from build123d import *

# Parameters (mm, degrees)
CHAMFER1_SIZE  = 0.79375
CHAMFER1_SIZE2 = 0.458271776
FILLET1_R      = 0.396875


with BuildPart() as part:
    # Sketch1 → Revolve1 (revolve)
    with BuildSketch(Plane.XY):
        Polygon((0, 0), (4.3561, 0), (4.3561, 22.225), (3.0607, 22.225), (3.0607, 24.60625), (3.4925, 24.60625), (3.4925, 38.1), (2.159, 38.1), (2.159, 2.273235175), (0, 2.273235175), align=None)
    revolve(axis=Axis((0, 0, 0), (0, 1, 0)))

    # Chamfer1
    chamfer1_edges = [part.edges().sort_by_distance(p)[0] for p in [
        (-3.4925, 38.1, 0),
    ]]
    chamfer1_side = [part.faces().sort_by_distance(p)[0] for p in [
        (-3.4925, 31.353125, 0),
    ]]
    chamfer(chamfer1_edges, length=CHAMFER1_SIZE, length2=CHAMFER1_SIZE2, reference=chamfer1_side[0])

    # Fillet1
    fillet1_edges = [part.edges().sort_by_distance(p)[0] for p in [
        (-3.0607, 24.60625, 0),
        (-3.0607, 22.225, 0),
    ]]
    fillet(fillet1_edges, radius=FILLET1_R)


solid = part.part
Can you work these out from the model? Positions are in its coordinate system, mm. A direction names the side the tool comes from. Round coordinates to 2 decimals unless told otherwise and drop trailing zeros. Order: outer loops, then holes, each group sorted by start corner. A loop starts at its lowest first (then second) coordinate and runs counter-clockwise, first axis right, second up. Notation, with made-up numbers: (18.5, -5.75) - (72.5, -5.75) arc R20 ccw to (72.5, 33.25) - close; hole circle Ø3 at (-28.5, -14). An arc over 180 degrees is marked (long way). Answer in a Markdown table with one row per item.
(1) Which directions (+Z, -Z, +X, -X, +Y, -Y) give clear straight access to the entire face, cutting with the end or side of a thin tool? Please do faces 1 (the face through (0, 0, 0)), 2 (the face through (0, 2.273, 0)), 3 (the face through (-0.66, 23.43, 2.99)).
From the geometry:
| item | result |
|---|---|
| face 1 | +Z, -Z, +X, -X, -Y |
| face 2 | +Y |
| face 3 | none |
(2) If we mould it in two halves opening along X, with no side actions, what happens to faces 4 (the face through (1.3, 38.1, 2)), 5 (the face through (-3.457, 11.268, 2.651)), 6 (the face through (-0.28, 19.94, -2.14))? For each: released by +X, released by -X, zero draft, split by the parting line, or undercut.
From the geometry:
| item | result |
|---|---|
| face 4 | zero draft |
| face 5 | split by the parting line |
| face 6 | undercut |
(3) Suppose I cut it at D-D, the plane y = 9. Please give me the cut outline in (x, z), plus the area to 3 significant figures.
From the geometry:
| item | result |
|---|---|
| outline | circle Ø8.71 at (0, 0); hole circle Ø4.32 at (0, 0) |
| area | 45.0 mm2 |
(4) Please list where these lines run through material, in increasing order: L1, parallel to X at y = 26, z = 0; L2, parallel to X at y = 13.5, z = 0. Write a range as from..to.
From the geometry:
| item | result |
|---|---|
| L1 | x = -3.49..-2.16, 2.16..3.49 |
| L2 | x = -4.36..-2.16, 2.16..4.36 |
(5) Suppose I cut it at B-B, the plane y = 27. Please give me the cut outline in (x, z) (1 decimal), plus the area to 3 significant figures.
From the geometry:
| item | result |
|---|---|
| outline | circle Ø7 at (0, 0); hole circle Ø4.3 at (0, 0) |
| area | 23.7 mm2 |
